```python
from build123d import *

# Parameters (mm, degrees)
F0_R     = 6.570466
F1_DEPTH = 20
F2_R     = 10
F3_R     = 10


with BuildPart() as f1:
    # F0 (on Front) → F1 (new body, symmetric)
    with BuildSketch(Plane.XZ):
        Polygon((-52.715916, 30.87929), (-52.715916, 0), (37.284084, 0), (37.284084, 5), (-47.715916, 5), (-47.715916, 30.87929), align=None)
        with BuildLine():
            Line((37.284084, 5), (37.284084, 0))
            Line((37.284084, 0), (80.273889, 0))
            Line((80.273889, 0), (80.273889, 20.87929))
            ThreePointArc((80.273889, 20.87929), (77.344957, 27.950358), (70.273889, 30.87929))
            Line((70.273889, 30.87929), (47.284084, 30.87929))
            ThreePointArc((47.284084, 30.87929), (40.213016, 27.950358), (37.284084, 20.87929))
            Line((37.284084, 20.87929), (37.284084, 5))
        make_face()
        with Locations((56.709491, 14.344878)):
            Circle(F0_R, mode=Mode.SUBTRACT)
    extrude(amount=F1_DEPTH, both=True)

    # F2
    f2_edges = [f1.edges().sort_by_distance(p)[0] for p in [
        (-50.215916, 20, 30.87929),
    ]]
    fillet(f2_edges, radius=F2_R)

    # F3
    f3_edges = [f1.edges().sort_by_distance(p)[0] for p in [
        (-50.215916, -20, 30.87929),
    ]]
    fillet(f3_edges, radius=F3_R)


solid = f1.part
```
Can you work these out from the model? Positions are in its coordinate system, mm. A direction names the side the tool comes from. Coordinates: 2 decimals unless noted, no trailing zeros. Order: outer loops, then holes, each group sorted by start corner. A loop starts at its lowest first (then second) coordinate and runs counter-clockwise, first axis right, second up.
1. Thinking about a two-plate mould opening in Z: for faces 1 (the face through (40.291, -0.28, 28.028)), 2 (the face through (51.495, 0.28, 10.347)), 3 (the face through (13, 0, 0)), which applies, +Z half, -Z half, draft (parallel to the pull), parting line (faces both ways), or undercut?
2. For faces 4 (the face through (-50.25, 16.99, 28.03)), 5 (the face through (-47.716, 0, 18)), 6 (the face through (-50.25, -16.99, 28.03)), which set-ups out of +Z, -Z, +X, -X, +Y, -Y let a thin tool reach every point of the face, with its end or its side?
3. If we section it at B-B (y = 11.5): Please give me the cut outline in (x, z).
4. If we section it at C-C (z = 27): Please give me the cut outline in (x, y).
5. I need wall thicknesses on line 1 (X direction, y = -15, z = 6); line 2 (X direction, y = 1.5, z = 10); line 3 (X direction, y = 1, z = 19.5). Which ranges of each line are inside material? Lowest first, please.
6. I'm going to push flat-ended pins straight in: pin 1 (1 mm diameter, centred on x = -9.5, y = -2.5, fed in from -Z); pin 2 (6 mm diameter, centred on x = 22.5, y = -7, fed in from +Z); pin 3 (10 mm diameter, centred on x = -10.5, z = 12, fed in from -Y). Where does each tip first touch, or does it pass through?
7. If we section it at D-D (z = 12): Please give me the cut outline in (x, y).
8. If we section it at A-A (x = 58.5): Please give me the cut outline in (y, z).
Entries:
1. face 1: +Z half
1. face 2: undercut
1. face 3: -Z half
2. face 4: +Z, -X, +Y
2. face 5: +Z, +Y, -Y
2. face 6: +Z, -X, -Y
3. outline: (-52.72, 0) - (80.27, 0) - (80.27, 20.88) arc R10 ccw to (70.27, 30.88) - (47.28, 30.88) arc R10 ccw to (37.28, 20.88) - (37.28, 5) - (-47.72, 5) - (-47.72, 30.77) - (-52.72, 30.77) - close; hole circle Ø13.14 at (56.71, 14.34)
4. outline: (-52.72, -17.91) - (-47.72, -17.91) - (-47.72, 17.91) - (-52.72, 17.91) - close; (39.38, -20) - (78.18, -20) - (78.18, 20) - (39.38, 20) - close
5. line 1: x = -52.72 to -47.72, 37.28 to 80.27
5. line 2: x = -52.72 to -47.72, 37.28 to 51.78, 61.64 to 80.27
5. line 3: x = -52.72 to -47.72, 37.28 to 52.64, 60.78 to 80.27
6. pin 1: stops at z = 0
6. pin 2: stops at z = 5
6. pin 3: passes through
7. outline: (-52.72, -20) - (-47.72, -20) - (-47.72, 20) - (-52.72, 20) - close; (37.28, -20) - (50.57, -20) - (50.57, 20) - (37.28, 20) - close; (62.85, -20) - (80.27, -20) - (80.27, 20) - (62.85, 20) - close
8. outline: (-20, 0) - (20, 0) - (20, 8.02) - (-20, 8.02) - close; (-20, 20.67) - (20, 20.67) - (20, 30.88) - (-20, 30.88) - close
